Part model, mm, in its own coordinate system. Face numbers are marked on the shaded views. Give positions to 0.01 mm unless a question says otherwise; leave off trailing zeros. Order: outer loops, then holes, each group sorted by start corner. A loop starts at its lowest first (then second) coordinate and runs counter-clockwise, first axis right, second up. Notation, with made-up numbers: (38.25, -34.75) -> (77.25, -34.75) arc R6 ccw to (77.25, -23.75) -> close; hole circle Ø5 at (34, -15). An arc over 180 degrees is marked (long way). Write item = value, one per line. Start each with the question number.
Item 1: Pull direction X, two halves, no side cores. Call the marked faces 1, 2, 3 and 4: +X half, -X half, draft (parallel to the pull), parting line (faces both ways), or undercut.
Item 2: Drill centre lines: line 1 along Z through (x, y) = (2.25, 4); line 2 along X through (y, z) = (8.5, 1.25); line 3 along Z through (x, y) = (16.5, 15.75). Where is each one in solid material? Low to high.
Item 3: Band-saw the part on A-A on x = 12.5. Write the cut outline in (y, z).
Item 4: Band-saw the part on B-B on y = 17.75. Write the cut outline in (x, z).
Item 5: Flat gauge pins, fed straight in: P1, Ø1.3, axis at x = 7.5, z = 2.5, coming from the +Y side; P2, Ø0.8, axis at y = 7, z = -0.5, coming from the -X side; P3, Ø0.8, axis at y = 9.5, z = -0.5, coming from the +X side. Where does each tip first touch, or does it go through?
Item 6: Band-saw the part on C-C on x = 16. Write the cut outline in (y, z).
Item 7: Band-saw the part on D-D on z = 2.25. Write the cut outline in (x, y), plus the area to 3 significant figures.
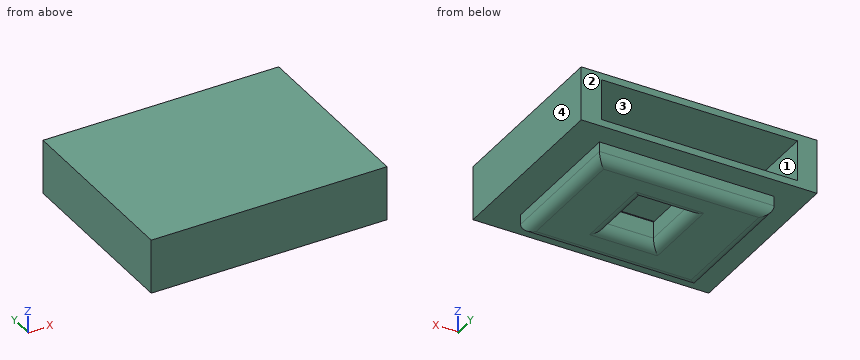
```python
from build123d import *

# Parameters (mm, degrees)
CROQUIS1_W              = 24.3
CROQUIS1_H              = 19.2
SALIENTE_EXTRUIR1_DEPTH = 5.6
CROQUIS2_W              = 20.2
CROQUIS2_H              = 4.2
CORTAR_EXTRUIR1_DEPTH   = 18
CROQUIS3_W              = 5
CROQUIS3_H              = 6.2
CORTAR_EXTRUIR2_DEPTH   = 2
CROQUIS5_W              = 18
CROQUIS5_H              = 14
CROQUIS5_W_2            = 5
CROQUIS5_H_2            = 6.2
SALIENTE_EXTRUIR3_DEPTH = 2
REDONDEO1_R             = 1


with BuildPart() as part:
    # Croquis1 → Saliente-Extruir1 (new body)
    with BuildSketch(Plane.XY):
        with Locations((12.15, 9.6)):
            Rectangle(CROQUIS1_W, CROQUIS1_H)
    extrude(amount=SALIENTE_EXTRUIR1_DEPTH)

    # Croquis2 → Cortar-Extruir1 (cut)
    with BuildSketch(Plane(origin=(0, 19.2, 0), x_dir=(1, 0, 0), z_dir=(0, 1, 0))):
        with Locations((12.1, -2.8)):
            Rectangle(CROQUIS2_W, CROQUIS2_H)
    extrude(amount=-CORTAR_EXTRUIR1_DEPTH, mode=Mode.SUBTRACT)

    # Croquis3 → Cortar-Extruir2 (cut)
    with BuildSketch(Plane(origin=(0, 0, 0), x_dir=(-1, 0, 0), z_dir=(0, 0, -1))):
        with Locations((-12.15, 9.9)):
            Rectangle(CROQUIS3_W, CROQUIS3_H)
    extrude(amount=-CORTAR_EXTRUIR2_DEPTH, mode=Mode.SUBTRACT)

    # Croquis5 → Saliente-Extruir3 (add)
    with BuildSketch(Plane(origin=(0, 0, 0), x_dir=(-1, 0, 0), z_dir=(0, 0, -1))):
        with Locations((-12.042477661, 9.840107479)):
            Rectangle(CROQUIS5_W, CROQUIS5_H)
        with Locations((-12.15, 9.9)):
            Rectangle(CROQUIS5_W_2, CROQUIS5_H_2, mode=Mode.SUBTRACT)
    extrude(amount=SALIENTE_EXTRUIR3_DEPTH)

    # Redondeo1
    redondeo1_edges = [part.edges().sort_by_distance(p)[0] for p in [
        (21.042477661, 9.840107479, -2),
        (12.042477661, 2.840107479, -2),
        (3.042477661, 9.840107479, -2),
        (12.042477661, 16.840107479, -2),
        (14.65, 9.9, -2),
        (12.15, 6.8, -2),
        (9.65, 9.9, -2),
        (12.15, 13, -2),
    ]]
    fillet(redondeo1_edges, radius=REDONDEO1_R)


solid = part.part
```
Values found:
q1.face_1 = undercut
q1.face_2 = draft
q1.face_3 = undercut
q1.face_4 = +X half
q2.line_1 = 0 to 0.7, 4.9 to 5.6
q2.line_2 = 0 to 2, 22.2 to 24.3
q2.line_3 = -2 to 0.7, 4.9 to 5.6
q3.outline = (0, 0) -> (2.84, 0) -> (2.84, -1) arc R1 ccw to (3.84, -2) -> (5.8, -2) arc R1 ccw to (6.8, -1) -> (6.8, 0.7) -> (1.2, 0.7) -> (1.2, 4.9) -> (19.2, 4.9) -> (19.2, 5.6) -> (0, 5.6) -> close; (13, -1) arc R1 ccw to (14, -2) -> (15.84, -2) arc R1 ccw to (16.84, -1) -> (16.84, 0) -> (19.2, 0) -> (19.2, 0.7) -> (13, 0.7) -> close
q4.outline = (0, 0) -> (24.3, 0) -> (24.3, 5.6) -> (0, 5.6) -> close; hole (2, 0.7) -> (22.2, 0.7) -> (22.2, 4.9) -> (2, 4.9) -> close
q5.P1 = 1.2
q5.P2 = 3.04
q5.P3 = 21.04
q6.outline = (0, 0) -> (2.84, 0) -> (2.84, -1) arc R1 ccw to (3.84, -2) -> (15.84, -2) arc R1 ccw to (16.84, -1) -> (16.84, 0) -> (19.2, 0) -> (19.2, 0.7) -> (1.2, 0.7) -> (1.2, 4.9) -> (19.2, 4.9) -> (19.2, 5.6) -> (0, 5.6) -> close
q7.outline = (0, 0) -> (24.3, 0) -> (24.3, 19.2) -> (22.2, 19.2) -> (22.2, 1.2) -> (2, 1.2) -> (2, 19.2) -> (0, 19.2) -> close
q7.area = 103 mm^2
